Source: three-view drawing plus pictorial views. Frame: mm from the lowest corner of the part. Round coordinates to 2 decimals unless told otherwise and drop trailing zeros. Order: outer loops, then holes, each group sorted by start corner. A loop starts at its lowest first (then second) coordinate and runs counter-clockwise, first axis right, second up. Notation, with made-up numbers: (-39, 63.25) -> (17, 63.25) arc R10 cw to (17, 72.25) -> close; hole circle Ø2 at (79.5, 50). An arc over 180 degrees is marked (long way). Answer as CSV lines item,"result".
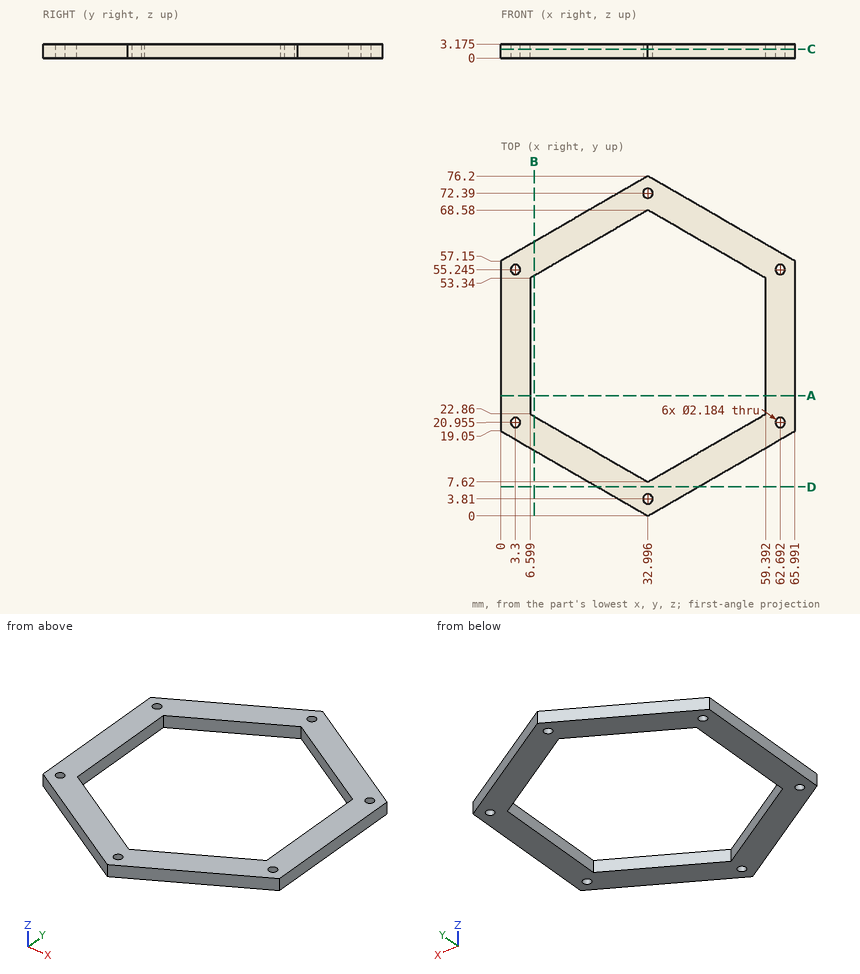
1. Pin query (flat end, axial travel): pin 1 (2 mm diameter, centred on x = 33, y = 3.81, fed in from -Z). Return the tip coordinate at first contact, or that it passes through.
Results below:
pin 1,"through"
2. Line query: L1, parallel to X at y = 26, z = 1.7; L2, parallel to X at y = 8.5, z = 3.05 (1 decimal); L3, parallel to Y at x = 33.5, z = 3. Output: solid intervals per line, ascending. Write a range as [from, to].
Results below:
L1,"[0, 6.6], [59.39, 65.99]"
L2,"[18.3, 31.5], [34.5, 47.7]"
L3,"[0.29, 2.84], [4.78, 7.91], [68.29, 71.42], [73.36, 75.91]"
3. Section query D-D on y = 6.5. Return loops of the section in (x, z) (1 decimal).
Results below:
outline,"(21.7, 0) -> (44.3, 0) -> (44.3, 3.2) -> (21.7, 3.2) -> close"
4. Section query B-B on x = 7.5. Return loops of the section in (y, z) (1 decimal).
Results below:
outline,"(14.7, 0) -> (22.3, 0) -> (22.3, 3.2) -> (14.7, 3.2) -> close; (53.9, 0) -> (61.5, 0) -> (61.5, 3.2) -> (53.9, 3.2) -> close"
5. Section query A-A on y = 27. Return loops of the section in (x, z) (1 decimal).
Results below:
outline,"(0, 0) -> (6.6, 0) -> (6.6, 3.2) -> (0, 3.2) -> close; (59.4, 0) -> (66, 0) -> (66, 3.2) -> (59.4, 3.2) -> close"
6. Section query C-C on z = 2.05. Give the number of separate pieces and of enclosed holes in the cut face.
Results below:
separate pieces,"1"
enclosed holes,"7"
